from build123d import *

# Parameters (mm, degrees)
F1_DEPTH = 38.1
F2_R     = 5.08
F3_R     = 5.08
F4_W     = 7.112
F4_H     = 25.4
F5_DEPTH = 38.1
F6_W     = 7.112
F6_H     = 25.4
F7_DEPTH = 7.112
F8_R     = 5.08


with BuildPart() as f1:
    # F0 (on Top) → F1 (new body)
    with BuildSketch(Plane.XY):
        with BuildLine():
            Line((0, 76.2), (0, 0))
            Line((0, 0), (6.35, 0))
            Line((6.35, 0), (6.35, 69.85))
            Line((6.35, 69.85), (38.1, 69.85))
            Line((38.1, 69.85), (38.1, 38.1))
            ThreePointArc((38.1, 38.1), (69.85, 7.30006), (101.6, 38.1))
            Line((101.6, 38.1), (95.25, 38.1))
            ThreePointArc((95.25, 38.1), (69.85, 13.646399), (44.45, 38.1))
            Line((44.45, 38.1), (44.45, 76.2))
            Line((44.45, 76.2), (0, 76.2))
        make_face()
    extrude(amount=F1_DEPTH)

    # F2
    f2_edges = [f1.edges().sort_by_distance(p)[0] for p in [
        (95.25, 38.1, 19.05),
    ]]
    fillet(f2_edges, radius=F2_R)

    # F3
    f3_edges = [f1.edges().sort_by_distance(p)[0] for p in [
        (44.45, 76.2, 19.05),
        (0, 76.2, 19.05),
    ]]
    fillet(f3_edges, radius=F3_R)

    # F4 (on face) → F5 (join)
    with BuildSketch(Plane(origin=(0, 0, 0), x_dir=(0, -1, 0), z_dir=(-1, 0, 0))):
        with Locations((-41.656, 19.05)):
            Rectangle(F4_W, F4_H)
    extrude(amount=F5_DEPTH)

    # F6 (on face) → F7 (join)
    with BuildSketch(Plane(origin=(0, 45.212, 0), x_dir=(-1, 0, 0), z_dir=(0, 1, 0))):
        with Locations((34.544, 19.05)):
            Rectangle(F6_W, F6_H)
    extrude(amount=F7_DEPTH)

    # F8
    f8_edges = [f1.edges().sort_by_distance(p)[0] for p in [
        (-15.494, 45.212, 31.75),
        (-15.494, 45.212, 6.35),
        (-30.988, 52.324, 19.05),
    ]]
    fillet(f8_edges, radius=F8_R)


solid = f1.part
Work out the finished part from the listing and answer in its coordinate system (mm). A direction names the side the tool comes from. Round coordinates to 2 decimals unless told otherwise and drop trailing zeros. Write each loop counter-clockwise with the first axis right and the second up, starting at its lowest first coordinate (ties: lowest second). Pieces come first, ordered by that corner, then holes. Notation, with made-up numbers: M 43.5,69.5 L 60.5,69.5 A14 ccw 60.5,82.5 Z; hole C 50.5,2.5 d8. An arc over 180 degrees is marked long. Use a Markdown table: item, result.
1) Consider line 1 (X direction, y = 45.5, z = 24.5); line 2 (X direction, y = 64.5, z = 10); line 3 (X direction, y = 20, z = 6). Determine where each line is inside the solid, lowest interval first. Write a range as [from, to].
Taken from the geometry:
| item | result |
|---|---|
| line 1 | x = [-38.1, -30.99], [0, 6.35], [38.1, 44.45] |
| line 2 | x = [0, 6.35], [38.1, 44.45] |
| line 3 | x = [0, 6.35], [44.44, 53.04], [86.66, 95.26] |
2) The part is cut by section D-D on x = 69.85. Give the vertices of the cut face in (y, z).
Taken from the geometry:
| item | result |
|---|---|
| outline | M 7.3,0 L 13.65,0 L 13.65,38.1 L 7.3,38.1 Z |
3) Determine the mould class of faces 5 (the face through (44.45, 54, 19)), 6 (the face through (1.528, 74.751, 19.317)), 7 (the face through (-26, 39.9, 6.35)), 8 (the face through (38.1, 54, 19)) for opening direction X: pulls with the +X half, pulls with the -X half, needs draft (parallel to the pull), parting line crosses it, or undercut.
Taken from the geometry:
| item | result |
|---|---|
| face 5 | pulls with the +X half |
| face 6 | pulls with the -X half |
| face 7 | needs draft |
| face 8 | undercut |
4) Which of the six approach directions +Z, -Z, +X, -X, +Y, -Y give full straight-line access (tool end or side, diameter ignored) to faces 1 (the face through (-32.44, 50.8, 19.23)), 2 (the face through (39, 38, 38.1)), 3 (the face through (-19, 38.1, 19)), 4 (the face through (22, 69.85, 19))?
Taken from the geometry:
| item | result |
|---|---|
| face 1 | +Z, -Z, +Y |
| face 2 | +Z, +X, -X, +Y, -Y |
| face 3 | +Z, -Z, -X, -Y |
| face 4 | +Z, -Z, -Y |
5) Flat-ended cylindrical pins translate along their axes: pin 1 (1 mm diameter, centred on x = -15, z = 12, fed in from -Y); pin 2 (15.5 mm diameter, centred on x = -12, y = 44, fed in from +Z); pin 3 (10 mm diameter, centred on y = 54.5, z = 6.5, fed in from +X); pin 4 (12 mm diameter, centred on y = 35, z = 13.5, fed in from +X). Find the tip coordinate at first contact, or state that the pin passes through.
Taken from the geometry:
| item | result |
|---|---|
| pin 1 | stops at y = 38.1 |
| pin 2 | stops at z = 31.75 |
| pin 3 | stops at x = 44.45 |
| pin 4 | stops at x = 101.6 |
6) The part is cut by section A-A on y = 56. Give the vertices of the cut face in (x, z), plus the area to 3 significant figures.
Taken from the geometry:
| item | result |
|---|---|
| outline | M 0,0 L 6.35,0 L 6.35,38.1 L 0,38.1 Z; M 38.1,0 L 44.45,0 L 44.45,38.1 L 38.1,38.1 Z |
| area | 484 mm2 |
7) The part is cut by section C-C on y = 15. Give the vertices of the cut face in (x, z).
Taken from the geometry:
| item | result |
|---|---|
| outline | M 0,0 L 6.35,0 L 6.35,38.1 L 0,38.1 Z; M 49.12,0 L 61.67,0 L 61.67,38.1 L 49.12,38.1 Z; M 78.03,0 L 90.58,0 L 90.58,38.1 L 78.03,38.1 Z |
